Model file for the job. Use its own axes, mm. Round coordinates to 2 decimals unless told otherwise and drop trailing zeros. Order: outer loops, then holes, each group sorted by start corner. A loop starts at its lowest first (then second) coordinate and runs counter-clockwise, first axis right, second up. Notation, with made-up numbers: (88, 53) -> (96, 53) arc R19 ccw to (96, 69) -> close; hole circle Ø2 at (80.25, 42). An arc over 180 degrees is marked (long way). Put each result on its own line as item: value. Start each with the question number.
Q1. Cut at B-B, the plane x = 2.3. State how many separate pieces and enclosed holes the cut face has, and give its area (3 significant figures).
Q2. Cut at A-A, the plane z = 129. List the corners of the cut face in (x, y) (3 decimals).
Q3. Flat gauge pins, fed straight in: P1, Ø4, axis at y = 85.35, z = -145, coming from the +X side (3 decimals); P2, Ø3, axis at y = 65.35, z = 155, coming from the +X side; P3, Ø5.5, axis at y = 8.175, z = -135, coming from the -X side; P4, Ø5.5, axis at y = 75.35, z = 155, coming from the +X side (3 decimals). Where does each tip first touch, or does it go through?
Q4. Cut at C-C, the plane z = -74.5. List the corners of the cut face in (x, y) (3 decimals), and give its area (4 significant figures).
Q5. Probe L1, parallel to Y at x = 1.05, z = -145 (3 decimals); L2, parallel to Y at x = 1, z = 155; L3, parallel to Z at x = 2.6, y = 52. List the from-to ranges inside material, lowest first.
from build123d import *

# Parameters (mm, degrees)
BOSS_EXTRUDE1_DEPTH                             = 3.175
CSK_FOR_M3_FLAT_HEAD_MACHINE_SCREW1_D           = 3.4
CSK_FOR_M3_FLAT_HEAD_MACHINE_SCREW1_CSINK_D     = 6.3
CSK_FOR_M3_FLAT_HEAD_MACHINE_SCREW1_CSINK_ANGLE = 90
SKETCH4_R                                       = 5
CUT_EXTRUDE1_DEPTH                              = 4.175
CSK_FOR_M3_FLAT_HEAD_MACHINE_SCREW2_D           = 3.4
CSK_FOR_M3_FLAT_HEAD_MACHINE_SCREW2_CSINK_D     = 6.3
CSK_FOR_M3_FLAT_HEAD_MACHINE_SCREW2_CSINK_ANGLE = 90
CSK_FOR_M3_FLAT_HEAD_MACHINE_SCREW3_D           = 3.4
CSK_FOR_M3_FLAT_HEAD_MACHINE_SCREW3_CSINK_D     = 6.3
CSK_FOR_M3_FLAT_HEAD_MACHINE_SCREW3_CSINK_ANGLE = 90
LPATTERN1_COUNT                                 = 2
LPATTERN1_PITCH                                 = 258


with BuildPart() as part:
    # Sketch1 → Boss-Extrude1 (new body)
    with BuildSketch(Plane(origin=(0, 0, 0), x_dir=(0, 0, -1), z_dir=(1, 0, 0))):
        Polygon((160, 0), (160, 3.175), (160, 47.175), (160, 50.35), (160, 60.35), (160, 90.35), (-160, 90.35), (-160, 60.35), (-160, 50.35), (-160, 47.175), (-160, 3.175), (-160, 0), align=None)
    extrude(amount=BOSS_EXTRUDE1_DEPTH)

    # CSK for M3 Flat Head Machine Screw1 (through all)
    with Locations(Plane(origin=(3.175, 0, 0), x_dir=(0, 0, -1), z_dir=(1, 0, 0))):
        with Locations((-145, 8.175), (-135, 8.175), (-105, 8.175), (-145, 55.35), (-135, 55.35), (-105, 55.35), (-145, 85.35), (-135, 85.35), (-5, 85.35)):
            csk_for_m3_flat_head_machine_screw1 = CounterSinkHole(CSK_FOR_M3_FLAT_HEAD_MACHINE_SCREW1_D / 2, CSK_FOR_M3_FLAT_HEAD_MACHINE_SCREW1_CSINK_D / 2, counter_sink_angle=CSK_FOR_M3_FLAT_HEAD_MACHINE_SCREW1_CSINK_ANGLE)

    # Mirror1: CSK for M3 Flat Head Machine Screw1 across plane
    add(csk_for_m3_flat_head_machine_screw1.mirror(Plane.XY), mode=Mode.SUBTRACT)

    # Sketch4 → Cut-Extrude1 (cut, through all)
    with BuildSketch(Plane(origin=(3.175, 0, 0), x_dir=(0, 0, -1), z_dir=(1, 0, 0))):
        with Locations((-129, 25.675)):
            Circle(SKETCH4_R)
        with Locations((129, 25.675)):
            Circle(SKETCH4_R)
        with BuildLine():
            Line((-100, 57.35), (-100, 0))
            Line((-100, 0), (100, 0))
            Line((100, 0), (100, 57.35))
            ThreePointArc((100, 57.35), (99.121320344, 59.471320344), (97, 60.35))
            Line((97, 60.35), (-97, 60.35))
            ThreePointArc((-97, 60.35), (-99.121320344, 59.471320344), (-100, 57.35))
        make_face()
    extrude(amount=-CUT_EXTRUDE1_DEPTH, mode=Mode.SUBTRACT)

    # CSK for M3 Flat Head Machine Screw2 (through all)
    with Locations(Plane(origin=(3.175, 0, 0), x_dir=(0, 0, -1), z_dir=(1, 0, 0))):
        with Locations((-155, 65.35), (-155, 75.35)):
            CounterSinkHole(CSK_FOR_M3_FLAT_HEAD_MACHINE_SCREW2_D / 2, CSK_FOR_M3_FLAT_HEAD_MACHINE_SCREW2_CSINK_D / 2, counter_sink_angle=CSK_FOR_M3_FLAT_HEAD_MACHINE_SCREW2_CSINK_ANGLE)

    # CSK for M3 Flat Head Machine Screw3 (through all)
    with Locations(Plane(origin=(3.175, 0, 0), x_dir=(0, 0, -1), z_dir=(1, 0, 0))):
        with Locations((-116.5, 31.175), (-135.25, 20.349682453), (-135.25, 42.000317547)):
            csk_for_m3_flat_head_machine_screw3 = CounterSinkHole(CSK_FOR_M3_FLAT_HEAD_MACHINE_SCREW3_D / 2, CSK_FOR_M3_FLAT_HEAD_MACHINE_SCREW3_CSINK_D / 2, counter_sink_angle=CSK_FOR_M3_FLAT_HEAD_MACHINE_SCREW3_CSINK_ANGLE)

    # LPattern1: CSK for M3 Flat Head Machine Screw3 ×2
    with Locations(*[(0, 0, -i * LPATTERN1_PITCH) for i in range(1, LPATTERN1_COUNT)]):
        add(csk_for_m3_flat_head_machine_screw3, mode=Mode.SUBTRACT)


solid = part.part
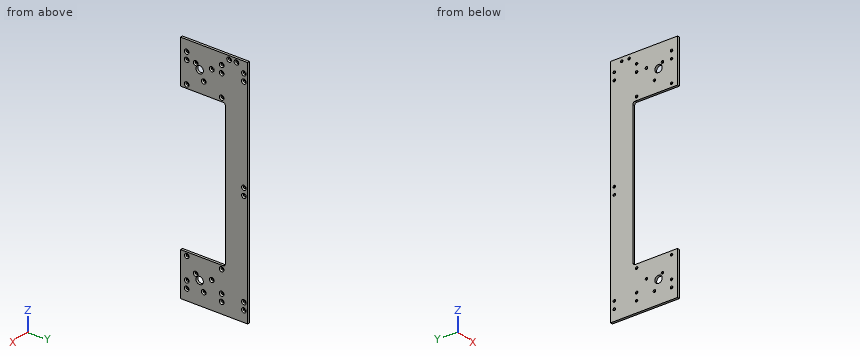
Ans:
1. separate pieces: 1
1. enclosed holes: 28
1. area: 16,300 mm^2
2. outline: (0, 0) -> (3.175, 0) -> (3.175, 20.675) -> (0, 20.675) -> close; (0, 30.675) -> (3.175, 30.675) -> (3.175, 90.35) -> (0, 90.35) -> close
3. P1: stops at x = 2.025
3. P2: passes through
3. P3: stops at x = 0
3. P4: stops at x = 2.775
4. outline: (0, 60.35) -> (3.175, 60.35) -> (3.175, 90.35) -> (0, 90.35) -> close
4. area: 95.25 mm^2
5. L1: y = 0 to 6.475, 9.875 to 53.65, 57.05 to 83.65, 87.05 to 90.35
5. L2: y = 0 to 63.65, 67.05 to 73.65, 77.05 to 90.35
5. L3: z = -160 to -100, 100 to 160
